Input: dimensioned drawing with shaded views. Units: mm. Origin: part minimum x, y, z. A direction names the side the tool comes from. Round coordinates to 2 decimals unless told otherwise and drop trailing zeros. Loops run counter-clockwise (first coordinate to the right, second up) from the corner with the lowest first, then second, coordinate; pieces in that order, holes last. Notation, with made-up numbers: M 51,34.5 L 83,34.5 A13 cw 83,40.5 Z; hole C -19.75,56 d9. An arc over 180 degrees is marked long. Put each result on its own line as item: value. Start each with the question number.
1) Pin query (flat end, axial travel): pin 1 (0.5 mm diameter, centred on x = 6, z = 7.5, fed in from +Y); pin 2 (1.5 mm diameter, centred on x = 14.5, y = 2, fed in from +Z); pin 3 (0.8 mm diameter, centred on x = 16, z = 7.5, fed in from -Y). Return the tip coordinate at first contact, or that it passes through.
2) Section B-B on y = 15.5. Output: boundary loops of the cut face in (x, z).
3) Section D-D on x = 19. Output: boundary loops of the cut face in (y, z).
4) Reachability of the marked faces 4 and 5 from +Z, -Z, +X, -X, +Y, -Y: full face, straight path, thin tool, end or side. Return the list, or none.
5) Line query: probe 1 along Y at (x, z) = (10, 4.75); probe 2 along Z at (x, y) = (15, 2.5); probe 3 along X at (y, z) = (3.75, 0.5). Output: solid intervals per line, ascending.
6) Section C-C on z = 3.25. Output: boundary loops of the cut face in (x, y).
7) Section A-A on x = 10. Output: boundary loops of the cut face in (y, z), plus the area to 3 significant figures.
8) Draft query along Y for the marked faces 1, 2 and 3. Return one class per face: +Y half, -Y half, draft (parallel to the pull), parting line (faces both ways), or undercut.
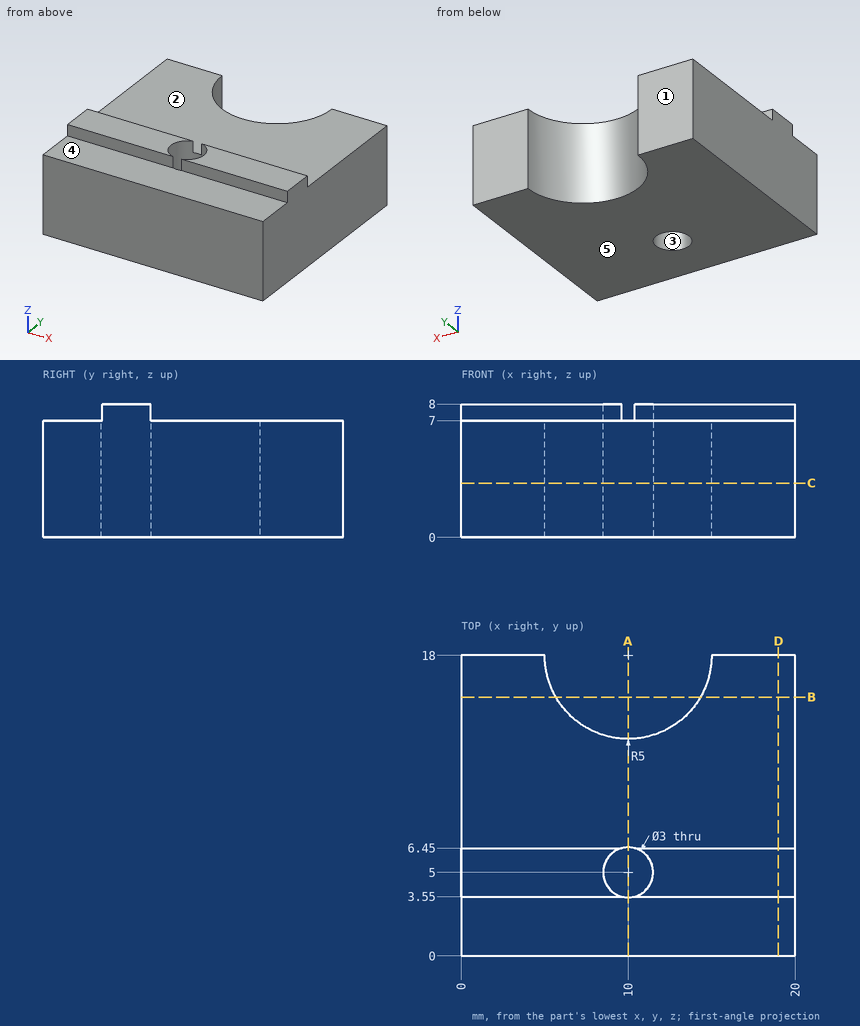
Geometry results:
1. pin 1: stops at y = 6.45
1. pin 2: stops at z = 7
1. pin 3: stops at y = 3.55
2. outline: M 0,0 L 5.67,0 L 5.67,7 L 0,7 Z; M 14.33,0 L 20,0 L 20,7 L 14.33,7 Z
3. outline: M 0,0 L 18,0 L 18,7 L 6.45,7 L 6.45,8 L 3.55,8 L 3.55,7 L 0,7 Z
4. face 4: +Z, +X, -X, -Y
4. face 5: -Z, +X, -X, +Y, -Y
5. probe 1: y = 0 to 3.5, 6.5 to 13
5. probe 2: z = 0 to 7
5. probe 3: x = 0 to 9.17, 10.83 to 20
6. outline: M 0,0 L 20,0 L 20,18 L 15,18 A5 cw 5,18 L 0,18 Z; hole C 10,5 d3
7. outline: M 0,0 L 3.5,0 L 3.5,7 L 0,7 Z; M 6.5,0 L 13,0 L 13,7 L 6.5,7 Z
7. area: 70.0 mm²
8. face 1: +Y half
8. face 2: draft
8. face 3: undercut
